Geometry check sheet. Reference: drawing and pictorial views, mm from the part's lowest x, y, z. Coordinates: 2 decimals unless noted, no trailing zeros. Write each loop counter-clockwise with the first axis right and the second up, starting at its lowest first coordinate (ties: lowest second). Pieces come first, ordered by that corner, then holes.
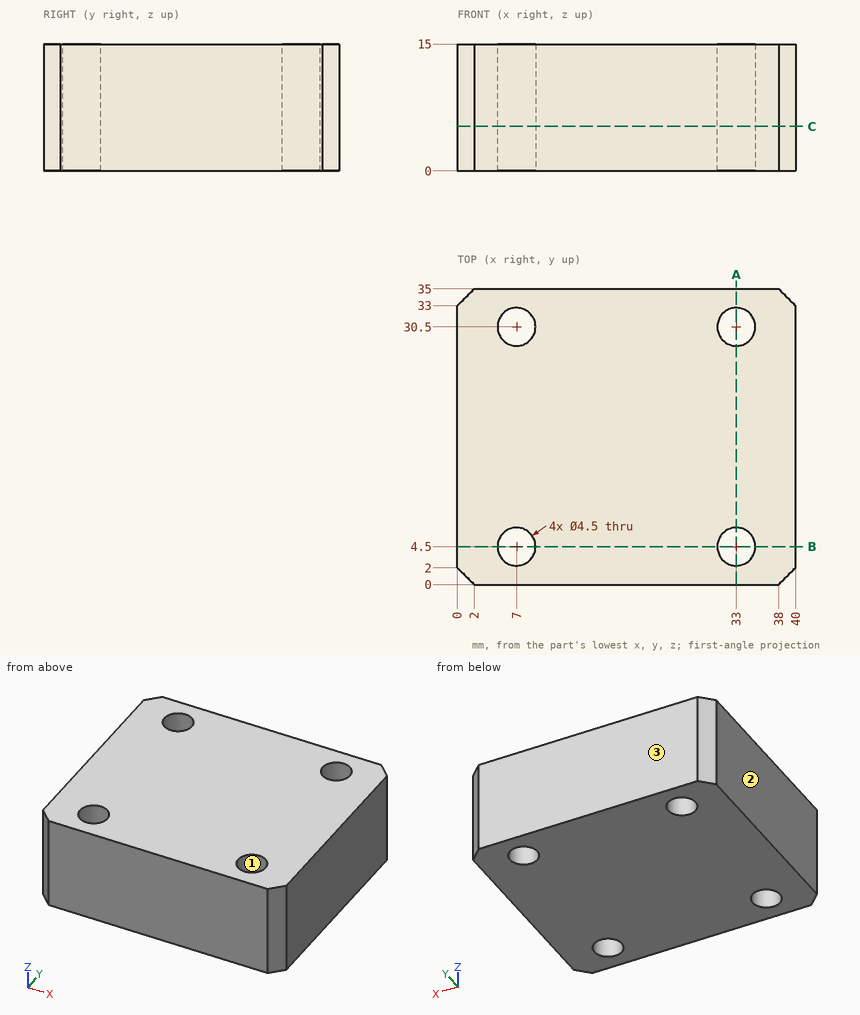
1. Sectioned sample at B-B, the plane y = 4.5. Record the boundary of the cut face in (x, z).
2. Material ranges on L1, parallel to Y at x = 33, z = 7.25; L2, parallel to X at y = 5, z = 10.5; L3, parallel to Y at x = 8, z = 11.75, recorded low to high.
3. Sectioned sample at A-A, the plane x = 33. Record the boundary of the cut face in (y, z), and give its area (3 significant figures).
4. Sectioned sample at C-C, the plane z = 5.25. Record the boundary of the cut face in (x, y).
5. Draft check along X on the marked faces 1, 2 and 3. Enter one of: pulls with the +X half, pulls with the -X half, needs draft (parallel to the pull), parting line crosses it, or undercut.
6. Gauge pin test, flat end, axial feed: P1, Ø4, axis at x = 7, y = 4.5, coming from the -Z side. Record the tip position at first contact, or that the pin passes through.
Outcome:
1. outline: (0, 0) - (4.75, 0) - (4.75, 15) - (0, 15) - close; (9.25, 0) - (30.75, 0) - (30.75, 15) - (9.25, 15) - close; (35.25, 0) - (40, 0) - (40, 15) - (35.25, 15) - close
2. L1: y = 0 to 2.25, 6.75 to 28.25, 32.75 to 35
2. L2: x = 0 to 4.81, 9.19 to 30.81, 35.19 to 40
2. L3: y = 0 to 2.48, 6.52 to 28.48, 32.52 to 35
3. outline: (0, 0) - (2.25, 0) - (2.25, 15) - (0, 15) - close; (6.75, 0) - (28.25, 0) - (28.25, 15) - (6.75, 15) - close; (32.75, 0) - (35, 0) - (35, 15) - (32.75, 15) - close
3. area: 390 mm2
4. outline: (0, 2) - (2, 0) - (38, 0) - (40, 2) - (40, 33) - (38, 35) - (2, 35) - (0, 33) - close; hole circle Ø4.5 at (7, 4.5); hole circle Ø4.5 at (7, 30.5); hole circle Ø4.5 at (33, 4.5); hole circle Ø4.5 at (33, 30.5)
5. face 1: undercut
5. face 2: pulls with the -X half
5. face 3: needs draft
6. P1: passes through
